Here's how the part is built. I have some questions about the finished solid (model axes, mm). Face numbers are marked on the shaded views. A direction names the side the tool comes from. Round coordinates to 2 decimals unless told otherwise and drop trailing zeros. Order: outer loops, then holes, each group sorted by start corner. A loop starts at its lowest first (then second) coordinate and runs counter-clockwise, first axis right, second up. Notation, with made-up numbers: M 6.5,14.25 L 65.5,14.25 A10 ccw 65.5,25.25 Z; hole C 66,74.5 d10. An arc over 180 degrees is marked long. Answer as CSV lines item,"result". Start each with the question number.
```python
from build123d import *

# Parameters (mm, degrees)
F1_W     = 101.6
F1_H     = 101.6
F2_DEPTH = 50.8
F3_W     = 101.6
F3_H     = 101.6
F4_DEPTH = 101.6
F5_W     = 101.6
F5_H     = 101.6
F6_DEPTH = 101.6
F7_W     = 101.6
F7_H     = 101.6
F8_DEPTH = 101.6


# Not quite as in the source:
# - a variable given as a bare number and used for a length is read in inches; the dataset says mm whatever the document's units were


with BuildPart() as f2:
    # F1 (on Front) → F2 (new body, symmetric)
    with BuildSketch(Plane.XZ):
        Rectangle(F1_W, F1_H)
    extrude(amount=F2_DEPTH, both=True)

    # F3 (on face) → F4 (join)
    with BuildSketch(Plane.XZ.offset(50.8)):
        Rectangle(F3_W, F3_H)
    extrude(amount=F4_DEPTH)

    # F5 (on face) → F6 (join)
    with BuildSketch(Plane.YZ.offset(50.8)):
        with Locations((-101.6, 0)):
            Rectangle(F5_W, F5_H)
    extrude(amount=F6_DEPTH)

    # F7 (on face) → F8 (join)
    with BuildSketch(Plane.XY.offset(50.8)):
        with Locations((0, -101.6)):
            Rectangle(F7_W, F7_H)
    extrude(amount=F8_DEPTH)


solid = f2.part
```
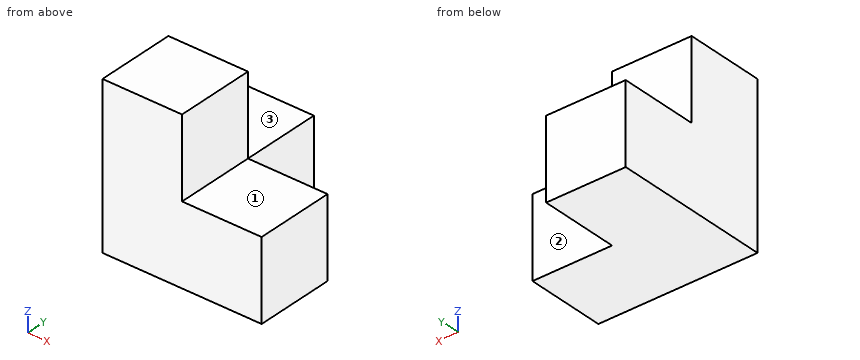
Item 1: If we section it at B-B on z = 41.5: Please give me the cut outline in (x, y).
Item 2: If we section it at C-C on y = -6: Please give me the cut outline in (x, z), and give its area (3 significant figures).
Item 3: For P1, Ø10, axis at x = 130.5, z = 57, coming from the +Y side; P2, Ø5, axis at x = 95, z = 35.5, coming from the +Y side, each with a flat end and sliding along its axis, tell me the tip position at first contact or that it passes through.
Item 4: If I drill on line 1 along Z through (x, y) = (62.5, -134); line 2 along Y through (x, z) = (8, 81), over which ranges is the centre line in solid material (lowest first)?
Item 5: If we section it at A-A on x = -18: Please give me the cut outline in (y, z).
Item 6: Which directions (+Z, -Z, +X, -X, +Y, -Y) give clear straight access to the entire face, cutting with the end or side of a thin tool? Please do the marked faces 1, 2 and 3.
Item 7: If we section it at D-D on x = 63.5: Please give me the cut outline in (y, z), and give its area (3 significant figures).
Geometry says:
1,outline,"M -50.8,-152.4 L 152.4,-152.4 L 152.4,-50.8 L 50.8,-50.8 L 50.8,50.8 L -50.8,50.8 Z"
2,outline,"M -50.8,-50.8 L 50.8,-50.8 L 50.8,50.8 L -50.8,50.8 Z"
2,area,"10,300 mm²"
3,P1,"through"
3,P2,"y = -50.8"
4,line 1,"-50.8 to 50.8"
4,line 2,"-152.4 to -50.8"
5,outline,"M -152.4,-50.8 L 50.8,-50.8 L 50.8,50.8 L -50.8,50.8 L -50.8,152.4 L -152.4,152.4 Z"
6,face 1,"+Z, +X, +Y, -Y"
6,face 2,"+Z, -Z, +X, +Y"
6,face 3,"+Z, +X, -X, +Y"
7,outline,"M -152.4,-50.8 L -50.8,-50.8 L -50.8,50.8 L -152.4,50.8 Z"
7,area,"10,300 mm²"
